Can you work these out from the model? Positions are in its coordinate system, mm. A direction names the side the tool comes from. Round coordinates to 2 decimals unless told otherwise and drop trailing zeros. Write each loop counter-clockwise with the first axis right and the second up, starting at its lowest first coordinate (ties: lowest second). Pieces come first, ordered by that corner, then holes.
Q1. If we section it at A-A (z = 8): Please give me the cut outline in (x, y), plus the area to 3 significant figures.
Q2. If we section it at B-B (y = 3.25): Give the number of separate pieces and of enclosed holes in the cut face, plus the area to 3 significant figures.
Q3. If we section it at D-D (y = 12.5): Please give me the cut outline in (x, z), plus the area to 3 significant figures.
Q4. Please list where these lines run through material, in increasing order: line 1 along Z through (x, y) = (1.35, 12.5); line 2 along Y through (x, z) = (3.25, -4.5); line 3 along Z through (x, y) = (3, 13.5).
Q5. If we section it at C-C (x = 1): Please give me the cut outline in (y, z).
Q6. For faces 1 (the flat face through (10, 4, 16.1)), 2 (the flat face through (7, 2, 0)), 3 (the flat face through (6.7, 5, 0.4)), which set-ups out of +Z, -Z, +X, -X, +Y, -Y let a thin tool reach every point of the face, with its end or its side?
Q7. I'm going to push flat-ended pins straight in: pin 1 Ø3 at (y, z) = (11.5, 18.5) entering from +X; pin 2 Ø8 at (x, z) = (9.5, 9.5) entering from +Y; pin 3 Ø3 at (x, z) = (10, 19) entering from -Y; pin 4 Ø4.5 at (x, z) = (10, -19) entering from +Y. Where does each tip first touch, or does it pass through?
Q8. We'd pull the mould along Z, two halves only. Please class faces 4 (the flat face through (0, 6, 0)), 5 (the flat face through (4, 6, -25)), 6 (the cylindrical face through (2.5, 12.4, -15)), 7 (the flat face through (3.521, 15.023, 21.43)): +Z half, -Z half, draft (parallel to the pull), parting line (faces both ways), or undercut.
from build123d import *

# Parameters (mm, degrees)
PAD_DEPTH       = 25
SKETCH001_R     = 1.75
POCKET_DEPTH    = 5.001
POCKET001_DEPTH = 3
SKETCH003_R     = 1.75
SKETCH003_W     = 12
SKETCH003_H     = 26
POCKET002_DEPTH = 20.001
POCKET003_DEPTH = 3
FILLET_R        = 3.99
POCKET004_DEPTH = 5.001
CHAMFER_SIZE    = 4
FILLET001_R     = 4


with BuildPart() as part:
    # Sketch → Pad (new body, symmetric)
    with BuildSketch(Plane.XY):
        Polygon((0, 0), (15, 0), (15, 5), (5, 5), (5, 20), (0, 20), align=None)
    extrude(amount=PAD_DEPTH, both=True)

    # Sketch001 (on Face4 of Pad) → Pocket (cut, through all)
    with BuildSketch(Plane.YZ.offset(5)):
        with Locations((12.5, 20)):
            Circle(SKETCH001_R)
        with Locations((12.5, -20)):
            Circle(SKETCH001_R)
    extrude(amount=-POCKET_DEPTH, mode=Mode.SUBTRACT)

    # Sketch002 (on Face10 of Pocket) → Pocket001 (cut)
    with BuildSketch(Plane.YZ.offset(5)):
        Polygon((14.174316, 17.1), (15.848632, 20), (14.174316, 22.9), (10.825684, 22.9), (9.151368, 20), (10.825684, 17.1), align=None)
        Polygon((14.174316, -22.9), (15.848632, -20), (14.174316, -17.1), (10.825684, -17.1), (9.151368, -20), (10.825684, -22.9), align=None)
    extrude(amount=-POCKET001_DEPTH, mode=Mode.SUBTRACT)

    # Sketch003 (on Face1 of Pocket001) → Pocket002 (cut, through all)
    with BuildSketch(Plane.XZ):
        with Locations((10, 19)):
            Circle(SKETCH003_R)
        with Locations((10, -19)):
            Circle(SKETCH003_R)
        with Locations((13, 0)):
            Rectangle(SKETCH003_W, SKETCH003_H)
    extrude(amount=-POCKET002_DEPTH, mode=Mode.SUBTRACT)

    # Sketch004 (on Face12 of Pocket002) → Pocket003 (cut)
    with BuildSketch(Plane(origin=(0, 5, 0), x_dir=(-1, 0, 0), z_dir=(0, 1, 0))):
        Polygon((-6.651368, 19), (-8.325684, 21.9), (-11.674316, 21.9), (-13.348632, 19), (-11.674316, 16.1), (-8.325684, 16.1), align=None)
        Polygon((-6.651368, -19), (-8.325684, -16.1), (-11.674316, -16.1), (-13.348632, -19), (-11.674316, -21.9), (-8.325684, -21.9), align=None)
    extrude(amount=-POCKET003_DEPTH, mode=Mode.SUBTRACT)

    # Fillet
    fillet_edges = [part.edges().sort_by_distance(p)[0] for p in [
        (15, 2.5, -25),
        (15, 2.5, -13),
        (7, 2.5, -13),
        (7, 2.5, 13),
        (15, 2.5, 13),
        (15, 2.5, 25),
    ]]
    fillet(fillet_edges, radius=FILLET_R)

    # Sketch005 (on Face20 of Fillet) → Pocket004 (cut, through all)
    with BuildSketch(Plane.YZ.offset(5)):
        with BuildLine():
            ThreePointArc((17.5, 10), (12.5, 15), (7.5, 10))
            Line((7.5, 10), (7.5, -10))
            ThreePointArc((7.5, -10), (12.5, -15), (17.5, -10))
            Line((17.5, 10), (17.5, -10))
        make_face()
    extrude(amount=-POCKET004_DEPTH, mode=Mode.SUBTRACT)

    # Chamfer
    chamfer_edges = [part.edges().sort_by_distance(p)[0] for p in [
        (2.5, 20, -25),
        (2.5, 20, 25),
    ]]
    chamfer(chamfer_edges, length=CHAMFER_SIZE)

    # Fillet001
    fillet001_edges = [part.edges().sort_by_distance(p)[0] for p in [
        (2.5, 20, -21),
        (2.5, 20, 21),
        (2.5, 16, -25),
        (2.5, 16, 25),
    ]]
    fillet(fillet001_edges, radius=FILLET001_R)


solid = part.part
A:
1. outline: (0, 0) - (7, 0) - (7, 5) - (5, 5) - (5, 7.5) - (0, 7.5) - close; (0, 17.5) - (5, 17.5) - (5, 20) - (0, 20) - close
1. area: 60.0 mm2
2. separate pieces: 1
2. enclosed holes: 2
2. area: 477 mm2
3. outline: (0, -25) - (5, -25) - (5, -22.9) - (2, -22.9) - (2, -21.75) - (0, -21.75) - close; (0, -18.25) - (2, -18.25) - (2, -17.1) - (5, -17.1) - (5, -15) - (0, -15) - close; (0, 15) - (5, 15) - (5, 17.1) - (2, 17.1) - (2, 18.25) - (0, 18.25) - close; (0, 21.75) - (2, 21.75) - (2, 22.9) - (5, 22.9) - (5, 25) - (0, 25) - close
3. area: 51.2 mm2
4. line 1: z = -25 to -21.75, -18.25 to -15, 15 to 18.25, 21.75 to 25
4. line 2: y = 0 to 7.5, 17.5 to 20
4. line 3: z = -25 to -22.9, -17.1 to -14.9, 14.9 to 17.1, 22.9 to 25
5. outline: (0, -25) - (14.34, -25) arc R4 ccw to (17.17, -23.83) - (18.83, -22.17) arc R4 ccw to (20, -19.34) - (20, 19.34) arc R4 ccw to (18.83, 22.17) - (17.17, 23.83) arc R4 ccw to (14.34, 25) - (0, 25) - close; hole (7.5, -10) arc R5 ccw to (17.5, -10) - (17.5, 10) arc R5 ccw to (7.5, 10) - close; hole circle Ø3.5 at (12.5, -20); hole circle Ø3.5 at (12.5, 20)
6. face 1: +Y
6. face 2: +X, +Y, -Y
6. face 3: +Z, -Z, +X, +Y
7. pin 1: stops at x = 5
7. pin 2: stops at y = 5
7. pin 3: passes through
7. pin 4: stops at y = 2
8. face 4: draft
8. face 5: -Z half
8. face 6: undercut
8. face 7: undercut
